```python
from build123d import *

# Parameters (mm, degrees)
SKETCH001_W   = 94
SKETCH001_H   = 40
SKETCH001_R   = 1.5
SKETCH001_W_2 = 70
SKETCH001_H_2 = 31
PAD001_DEPTH  = 3
SKETCH002_W   = 79.5
SKETCH002_H   = 37.5
POCKET_DEPTH  = 1.5
FILLET_R      = 5
CHAMFER_SIZE  = 2


with BuildPart() as part:
    # Sketch001 → Pad001 (new body)
    with BuildSketch(Plane.XY):
        Rectangle(SKETCH001_W, SKETCH001_H)
        with Locations((-42.85, 15)):
            Circle(SKETCH001_R, mode=Mode.SUBTRACT)
        with Locations((-42.85, -15)):
            Circle(SKETCH001_R, mode=Mode.SUBTRACT)
        with Locations((42.85, 15)):
            Circle(SKETCH001_R, mode=Mode.SUBTRACT)
        with Locations((42.85, -15)):
            Circle(SKETCH001_R, mode=Mode.SUBTRACT)
        with Locations((2.75, 0)):
            Rectangle(SKETCH001_W_2, SKETCH001_H_2, mode=Mode.SUBTRACT)
    extrude(amount=PAD001_DEPTH)

    # Sketch002 (on Face13 of Pad001) → Pocket (cut)
    with BuildSketch(Plane(origin=(0, 0, 0), x_dir=(1, 0, 0), z_dir=(0, 0, -1))):
        Rectangle(SKETCH002_W, SKETCH002_H)
    extrude(amount=-POCKET_DEPTH, mode=Mode.SUBTRACT)

    # Fillet
    fillet_edges = [part.edges().sort_by_distance(p)[0] for p in [
        (-47, -20, 1.5),
        (-47, 20, 1.5),
        (47, -20, 1.5),
        (47, 20, 1.5),
    ]]
    fillet(fillet_edges, radius=FILLET_R)

    # Chamfer
    chamfer_edges = [part.edges().sort_by_distance(p)[0] for p in [
        (41.35, -15, 3),
        (41.35, 15, 3),
        (-44.35, -15, 3),
        (-44.35, 15, 3),
    ]]
    chamfer(chamfer_edges, length=CHAMFER_SIZE)


with BuildPart() as part_1:
    # Body001 placement: moved
    add(part.part.moved(Location((0, 5, 2))))


solid = part_1.part
```
Verification items for the finished model (mm, model axes). Coordinates: 2 decimals unless noted, no trailing zeros. Write each loop counter-clockwise with the first axis right and the second up, starting at its lowest first coordinate (ties: lowest second). Pieces come first, ordered by that corner, then holes. Notation, with made-up numbers: M -9,0.25 L 9,0.25 A18 ccw 9,23.25 Z; hole C -5,66 d11. An arc over 180 degrees is marked long. Answer as a JSON object with one key per item and string values. Group by question number.
(1) Cross-section at D-D, the plane x = -38.5. Record the cut outline in (y, z).
(2) Material ranges on line 1 (X direction, y = 3.5, z = 4.55); line 2 (Y direction, x = -42.85, z = 2.35); line 3 (X direction, y = 14.5, z = 2.4), recorded low to high.
(3) Release check for a two-part mould opening along Y. For faces 1 (the face through (-46, 23, 4)), 2 (the face through (-41.464, -10.575, 2.493)), 3 (the face through (-9, -12, 3.5)), 4 (the face through (0, 24, 2)) record: +Y half, -Y half, draft (parallel to the pull), parting line (faces both ways), or undercut.
(4) Gauge pin test, flat ends, axial feed: pin 1 (5 mm diameter, centred on x = 35.5, y = -9, fed in from -Z); pin 2 (2.5 mm diameter, centred on x = 42.85, y = 20, fed in from -Z); pin 3 (3.5 mm diameter, centred on x = -42.85, y = 20, fed in from +Z). Record the tip position at first contact, or that the pin passes through.
(5) Cross-section at A-A, the plane y = 15.5. Record the cut outline in (x, z).
(6) Cross-section at C-C, the plane x = 10.5. Record the cut outline in (y, z), and give its area (4 significant figures).
(7) Cross-section at B-B, the plane z = 4.2. Record the cut outline in (x, y).
Reply:
{
 "1": {"outline": "M -15,2 L -13.75,2 L -13.75,3.5 L 23.75,3.5 L 23.75,2 L 25,2 L 25,5 L -15,5 Z"},
 "2": {"line 1": "-47 to -32.25, 37.75 to 47", "line 2": "-14.93 to -11.5, -8.5 to 18.5, 21.5 to 24.93", "line 3": "-47 to -39.75, 39.75 to 47"},
 "3": {"face 1": "+Y half", "face 2": "undercut", "face 3": "undercut", "face 4": "draft"},
 "4": {"pin 1": "z = 3.5", "pin 2": "through", "pin 3": "z = 3.25"},
 "5": {"outline": "M -47,2 L -39.75,2 L -39.75,3.5 L -32.25,3.5 L -32.25,5 L -47,5 Z; M 37.75,3.5 L 39.75,3.5 L 39.75,2 L 47,2 L 47,5 L 37.75,5 Z"},
 "6": {"outline": "M -15,2 L -13.75,2 L -13.75,3.5 L -10.5,3.5 L -10.5,5 L -15,5 Z; M 20.5,3.5 L 23.75,3.5 L 23.75,2 L 25,2 L 25,5 L 20.5,5 Z", "area": "17.25 mm²"},
 "7": {"outline": "M -47,-10 A5 ccw -42,-15 L 42,-15 A5 ccw 47,-10 L 47,20 A5 ccw 42,25 L -42,25 A5 ccw -47,20 Z; hole C -42.85,-10 d5.4; hole C -42.85,20 d5.4; hole M -32.25,-10.5 L 37.75,-10.5 L 37.75,20.5 L -32.25,20.5 Z; hole C 42.85,-10 d5.4; hole C 42.85,20 d5.4"}
}
